Check sheet for the drawn part. Datum: minimum x, y, z corner. Units: mm. Round coordinates to 2 decimals unless told otherwise and drop trailing zeros. Write each loop counter-clockwise with the first axis right and the second up, starting at its lowest first coordinate (ties: lowest second). Pieces come first, ordered by that corner, then holes. Notation, with made-up numbers: (22.25, -31.75) -> (78.25, -31.75) arc R26 ccw to (78.25, -15.75) -> close; hole circle Ø7 at (82, -31). An arc over 180 degrees is marked (long way). One line per item, written item: value.
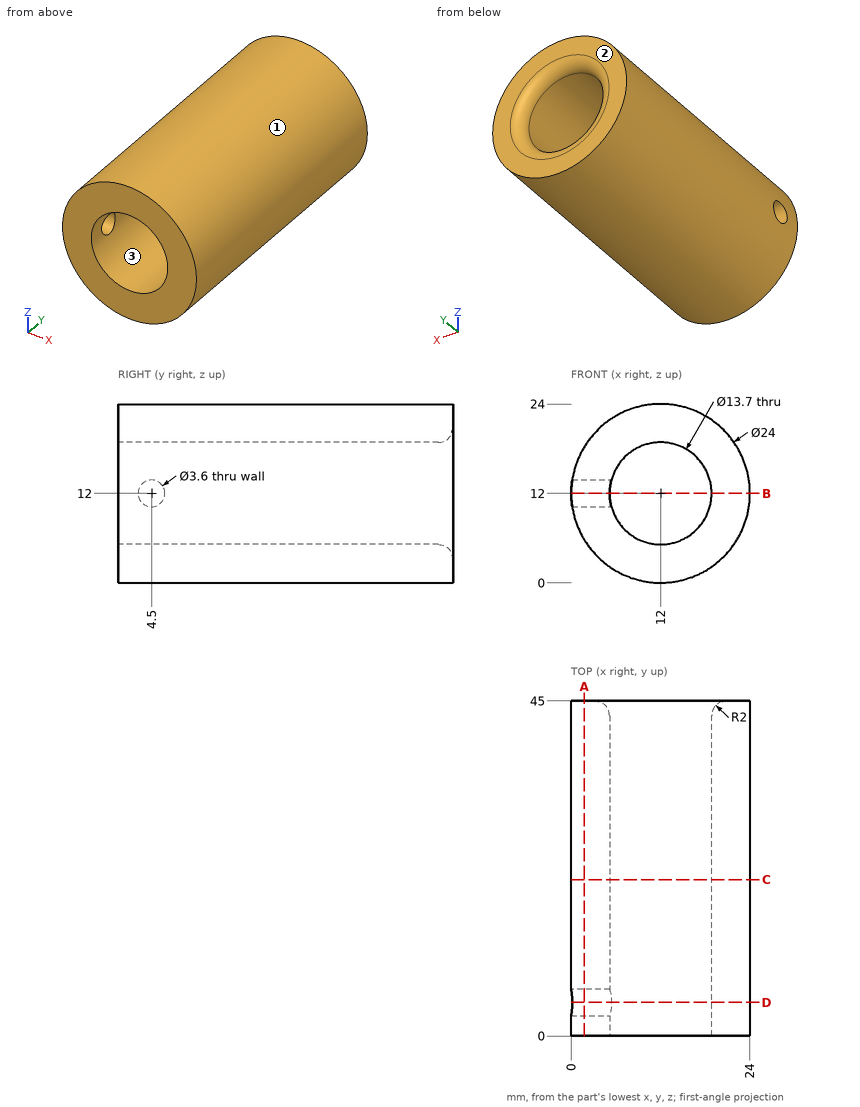
Item 1: Mould release check, pull along Z, two halves, no side actions. Record for the marked faces 1, 2 and 3: pulls with the +Z half, pulls with the -Z half, needs draft (parallel to the pull), parting line crosses it, or undercut.
Answer:
face 1: parting line crosses it
face 2: needs draft
face 3: undercut
Item 2: Sectioned sample at D-D on y = 4.5. Enter the section's corners in (x, z), and give its area (3 significant figures).
Answer:
outline: (0.14, 10.2) arc R12 ccw (long way) to (0.14, 13.8) -> (5.39, 13.8) arc R6.85 cw (long way) to (5.39, 10.2) -> close
area: 286 mm^2
Item 3: Depth check by flat-ended pin: P1, Ø12, axis at y = 26.5, z = 12.5, coming from the -X side; P2, Ø1, axis at y = 9, z = 4.5, coming from the +X side; P3, Ø8, axis at y = 14, z = 21, coming from the +X side; P4, Ø3, axis at y = 27.5, z = 18, coming from the +X side. Enter the tip coordinate at first touch or a pass-through.
Answer:
P1: stops at x = 0
P2: stops at x = 21.75
P3: stops at x = 22.91
P4: stops at x = 23.12
Item 4: Sectioned sample at A-A on x = 1.75. Enter the section's corners in (y, z), and give its area (3 significant figures).
Answer:
outline: (0, 5.76) -> (45, 5.76) -> (45, 18.24) -> (0, 18.24) -> close; hole circle Ø3.6 at (4.5, 12)
area: 551 mm^2
Item 5: Sectioned sample at C-C on y = 21. Enter the section's corners in (x, z).
Answer:
outline: circle Ø24 at (12, 12); hole circle Ø13.7 at (12, 12)
Item 6: Thickness scan on line 1 (Z direction, x = 12, y = 11.5); line 2 (Z direction, x = 10.5, y = 30); line 3 (X direction, y = 14, z = 8.75). Record the ranges inside material, lowest first.
Answer:
line 1: z = 0 to 5.15, 18.85 to 24
line 2: z = 0.09 to 5.32, 18.68 to 23.91
line 3: x = 0.45 to 5.97, 18.03 to 23.55
Item 7: Sectioned sample at B-B on z = 12. Count the separate pieces of the cut face and the enclosed holes in it, and give its area (3 significant figures).
Answer:
separate pieces: 3
enclosed holes: 0
area: 443 mm^2
